```python
from build123d import *

# Parameters (mm, degrees)
BOSS_EXTRUDE1_DEPTH               = 19.05
F_3_8_16_TAPPED_HOLE1_D           = 9.525
F_3_8_16_TAPPED_HOLE1_CSINK_D     = 10.795
F_3_8_16_TAPPED_HOLE1_CSINK_ANGLE = 90


with BuildPart() as part:
    # Sketch6 → Boss-Extrude1 (new body)
    with BuildSketch(Plane.XY):
        Polygon((-28.956, 57.404), (28.956, 57.404), (30.48, 55.88), (30.48, -10.922), (28.956, -12.446), (-28.956, -12.446), (-30.48, -10.922), (-30.48, 55.88), align=None)
        with BuildLine():
            Line((9.525, 4.9022), (18.415, 4.9022))
            ThreePointArc((18.415, 4.9022), (23.3172, 0), (18.415, -4.9022))
            Line((18.415, -4.9022), (9.525, -4.9022))
            ThreePointArc((9.525, -4.9022), (4.6228, 0), (9.525, 4.9022))
        make_face(mode=Mode.SUBTRACT)
        with BuildLine():
            Line((-9.525, 4.9022), (-18.415, 4.9022))
            ThreePointArc((-18.415, 4.9022), (-23.3172, 0), (-18.415, -4.9022))
            Line((-18.415, -4.9022), (-9.525, -4.9022))
            ThreePointArc((-9.525, -4.9022), (-4.6228, 0), (-9.525, 4.9022))
        make_face(mode=Mode.SUBTRACT)
    extrude(amount=-BOSS_EXTRUDE1_DEPTH)

    # 3/8-16 Tapped Hole1 (through all)
    with Locations(Plane.XY):
        with Locations((0, 45.5295)):
            CounterSinkHole(F_3_8_16_TAPPED_HOLE1_D / 2, F_3_8_16_TAPPED_HOLE1_CSINK_D / 2, counter_sink_angle=F_3_8_16_TAPPED_HOLE1_CSINK_ANGLE)


solid = part.part
```
Here's how the part is built. I have some questions about the finished solid (model axes, mm). A direction names the side the tool comes from. Round coordinates to 2 decimals unless told otherwise and drop trailing zeros. Loops run counter-clockwise (first coordinate to the right, second up) from the corner with the lowest first, then second, coordinate; pieces in that order, holes last. Notation, with made-up numbers: (83, -30.5) -> (100, -30.5) arc R7 cw to (100, -20.5) -> close; hole circle Ø3 at (70.5, 16). An arc over 180 degrees is marked (long way). Answer as CSV lines item,"result". Start each with the question number.
1. Imagine slicing it at B-B on x = -17.5. Write out the boundary of the cut face in (y, z), plus the area to 3 significant figures.
2. For faces 1 (the face through (0, 23, -19.05)), 2 (the face through (23.316, 0.108, -9.392)), which set-ups out of +Z, -Z, +X, -X, +Y, -Y let a thin tool reach every point of the face, with its end or its side?
3. I'm going to push a flat-ended pin straight in: P1, Ø8.5, axis at x = 0, y = 45.53, coming from the +Z side. Where does the tip first touch, or does it pass through?
4. Imagine slicing it at C-C on z = -4.25. Write out the boundary of the cut face in (x, y) (1 decimal).
5. If we mould it in two halves opening along Y, with no side actions, what happens to faces 3 (the face through (29.71, 56.65, -9.39)), 4 (the face through (-30.48, 22, -9)), 5 (the face through (14, -4.902, -9))? For each: pulls with the +Y half, pulls with the -Y half, needs draft (parallel to the pull), parting line crosses it, or undercut.
6. Imagine slicing it at D-D on x = 0. Write out the boundary of the cut face in (y, z) (3 decimals), plus the area to 3 significant figures.
7. Imagine slicing it at A-A on y = 0. Write out the boundary of the cut face in (x, z).
8. I need wall thicknesses on probe 1 along X at (y, z) = (0, -7.5); probe 2 along Y at (x, z) = (-14, -17.5); probe 3 along Y at (x, z) = (20, -15.5). Which ranges of each line are inside material? Lowest first, please. Write a range as from..to.
Solution:
1,outline,"(-12.45, -19.05) -> (-4.9, -19.05) -> (-4.9, 0) -> (-12.45, 0) -> close; (4.9, -19.05) -> (57.4, -19.05) -> (57.4, 0) -> (4.9, 0) -> close"
1,area,"1,140 mm²"
2,face 1,"-Z, +X, -X, +Y, -Y"
2,face 2,"+Z, -Z"
3,P1,"through"
4,outline,"(-30.5, -10.9) -> (-29, -12.4) -> (29, -12.4) -> (30.5, -10.9) -> (30.5, 55.9) -> (29, 57.4) -> (-29, 57.4) -> (-30.5, 55.9) -> close; hole (-18.4, -4.9) -> (-9.5, -4.9) arc R4.9 ccw to (-9.5, 4.9) -> (-18.4, 4.9) arc R4.9 ccw to start; hole circle Ø9.5 at (0, 45.5); hole (9.5, -4.9) -> (18.4, -4.9) arc R4.9 ccw to (18.4, 4.9) -> (9.5, 4.9) arc R4.9 ccw to start"
5,face 3,"pulls with the +Y half"
5,face 4,"needs draft"
5,face 5,"undercut"
6,outline,"(-12.446, -19.05) -> (40.767, -19.05) -> (40.767, -0.635) -> (40.132, 0) -> (-12.446, 0) -> close; (50.292, -19.05) -> (57.404, -19.05) -> (57.404, 0) -> (50.927, 0) -> (50.292, -0.635) -> close"
6,area,"1,150 mm²"
7,outline,"(-30.48, -19.05) -> (-23.32, -19.05) -> (-23.32, 0) -> (-30.48, 0) -> close; (-4.62, -19.05) -> (4.62, -19.05) -> (4.62, 0) -> (-4.62, 0) -> close; (23.32, -19.05) -> (30.48, -19.05) -> (30.48, 0) -> (23.32, 0) -> close"
8,probe 1,"-30.48..-23.32, -4.62..4.62, 23.32..30.48"
8,probe 2,"-12.45..-4.9, 4.9..57.4"
8,probe 3,"-12.45..-4.64, 4.64..57.4"
